Autodesk Inventor part; units mm, degrees
ref_plane "YZ Plane" through (0, 0, 0) normal (1, 0, 0) x (0, 1, 0)
ref_plane "XZ Plane" through (0, 0, 0) normal (0, 1, 0) x (-1, 0, 0)
ref_plane "XY Plane" through (0, 0, 0) normal (0, 0, 1) x (1, 0, 0)
sketch "Sketch1" plane through (0, 0, 0) normal (0, 1, 0) x (-1, 0, 0)
  circle A0 centre (0, 0) radius 2.75
  line L0 (2.75, -1.5877) -> (0, -3.1754)
  line L1 (0, -3.1754) -> (-2.75, -1.5877)
  line L2 (-2.75, -1.5877) -> (-2.75, 1.5877)
  line L3 (-2.75, 1.5877) -> (0, 3.1754)
  line L4 (0, 3.1754) -> (2.75, 1.5877)
  line L5 (2.75, 1.5877) -> (2.75, -1.5877)
  circle A1 centre (0, 0) radius 1.25
  point P0 (2.75, 0)
  dimension "d0" = 5.5
  dimension "d1" = 2.5
extrude "Extrusion1" add sketch "Sketch1" along normal blind 30
thread "Thread1"
properties part number "Distance_M3_30" material "Nickel-Copper Alloy 400"
The model under review builds one solid part; all positions refer to its coordinate system, in mm. Round coordinates to 2 decimals unless told otherwise and drop trailing zeros. Loops run counter-clockwise (first coordinate to the right, second up) from the corner with the lowest first, then second, coordinate; pieces in that order, holes last.
Item 1: For line 1 (Z direction, x = 0.9, y = 7); line 2 (X direction, y = 22, z = 0.25); line 3 (Z direction, x = 1, y = 12.5), list the stretches that pass through material, from the lowest coordinate up.
Determined:
line 1: z = -2.66 to -0.87, 0.87 to 2.66
line 2: x = -2.75 to -1.22, 1.22 to 2.75
line 3: z = -2.6 to -0.75, 0.75 to 2.6
Item 2: Take a section at C-C (x = 0.6). Write out the cut boundary in (y, z), then the cut area to 3 significant figures.
Determined:
outline: (0, -2.83) - (30, -2.83) - (30, -1.1) - (0, -1.1) - close; (0, 1.1) - (30, 1.1) - (30, 2.83) - (0, 2.83) - close
area: 104 mm2
Item 3: Take a section at B-B (z = -0.75). Write out the cut boundary in (x, y).
Determined:
outline: (-2.75, 0) - (-1, 0) - (-1, 30) - (-2.75, 30) - close; (1, 0) - (2.75, 0) - (2.75, 30) - (1, 30) - close
Item 4: Take a section at A-A (y = 8.25). Write out the cut boundary in (x, z).
Determined:
outline: (-2.75, -1.59) - (0, -3.18) - (2.75, -1.59) - (2.75, 1.59) - (0, 3.18) - (-2.75, 1.59) - close; hole circle Ø2.5 at (0, 0)
Item 5: Clearance check with flat-ended pins moving along their axes: pin 1 Ø3 at (x, z) = (0, 0) entering from -Y; pin 2 Ø2 at (x, y) = (-0.5, 23) entering from -Z. State where each tip first meets the part, or that it passes through.
Determined:
pin 1: stops at y = 0
pin 2: stops at z = -3.18
Item 6: Take a section at D-D (x = -1.75). Write out the cut boundary in (y, z).
Determined:
outline: (0, -2.17) - (30, -2.17) - (30, 2.17) - (0, 2.17) - close
